Could you check a few things on this model? Use its own coordinates, in mm. A direction names the side the tool comes from. Round coordinates to 2 decimals unless told otherwise and drop trailing zeros. Write each loop counter-clockwise with the first axis right and the second up, starting at its lowest first coordinate (ties: lowest second). Pieces come first, ordered by that corner, then holes. Notation, with made-up numbers: (35, 40) - (71, 40) arc R12 cw to (71, 46) - close; hole circle Ø9 at (-12.5, -7). An arc over 180 degrees is marked (long way). Put each result on its own line as item: value.
from build123d import *

# Parameters (mm, degrees)
F0_R     = 3
F0_R_2   = 5.25
F1_DEPTH = 2


with BuildPart() as f1:
    # F0 (on Top) → F1 (new body)
    with BuildSketch(Plane.XY):
        with BuildLine():
            Line((-106.994636, 73.57139), (-148.369657, 73.57139))
            ThreePointArc((-148.369657, 73.57139), (-171.369657, 19.821374), (-148.369657, -33.928643))
            Line((-148.369657, -33.928643), (-106.994636, -33.928643))
            ThreePointArc((-106.994636, -33.928643), (-97.994636, -30.928643), (-88.994636, -33.928643))
            Line((-88.994636, -33.928643), (-47.619614, -33.928643))
            ThreePointArc((-47.619614, -33.928643), (-24.619614, 19.821374), (-47.619614, 73.57139))
            Line((-47.619614, 73.57139), (-88.994636, 73.57139))
            ThreePointArc((-88.994636, 73.57139), (-97.994636, 70.57139), (-106.994636, 73.57139))
        make_face()
        with Locations((-144.276634, -8.428643)):
            Circle(F0_R, mode=Mode.SUBTRACT)
        with Locations((-127.869657, 19.821374)):
            Circle(F0_R_2, mode=Mode.SUBTRACT)
        with Locations((-68.119614, 19.821374)):
            Circle(F0_R_2, mode=Mode.SUBTRACT)
        with BuildLine():
            Line((-123.994636, 30.821374), (-123.994636, 57.321374))
            Line((-123.994636, 57.321374), (-71.994636, 57.321374))
            Line((-71.994636, 57.321374), (-71.994636, 30.821374))
            Line((-71.994636, 30.821374), (-77.983549, 27.821374))
            ThreePointArc((-77.983549, 27.821374), (-77.149435, 23.859964), (-76.869614, 19.821374))
            ThreePointArc((-76.869614, 19.821374), (-77.149435, 15.782783), (-77.983549, 11.821374))
            Line((-77.983549, 11.821374), (-71.994636, 8.821374))
            Line((-71.994636, 8.821374), (-71.994636, -17.678626))
            Line((-71.994636, -17.678626), (-123.994636, -17.678626))
            Line((-123.994636, -17.678626), (-123.994636, 8.821374))
            Line((-123.994636, 8.821374), (-118.005723, 11.821374))
            ThreePointArc((-118.005723, 11.821374), (-118.839837, 15.782783), (-119.119657, 19.821374))
            ThreePointArc((-119.119657, 19.821374), (-118.839837, 23.859964), (-118.005723, 27.821374))
            Line((-118.005723, 27.821374), (-123.994636, 30.821374))
        make_face(mode=Mode.SUBTRACT)
        with Locations((-144.276634, 48.07139)):
            Circle(F0_R, mode=Mode.SUBTRACT)
    extrude(amount=F1_DEPTH)


solid = f1.part
(1) Imagine slicing it at C-C, the plane z = 0.5. List the corners of the cut face in (x, y) for me.
Values found:
outline: (-148.37, -33.93) - (-106.99, -33.93) arc R15 cw to (-88.99, -33.93) - (-47.62, -33.93) arc R74.31 ccw to (-47.62, 73.57) - (-88.99, 73.57) arc R15 cw to (-106.99, 73.57) - (-148.37, 73.57) arc R74.31 ccw to start; hole circle Ø6 at (-144.28, -8.43); hole circle Ø6 at (-144.28, 48.07); hole circle Ø10.5 at (-127.87, 19.82); hole (-123.99, -17.68) - (-71.99, -17.68) - (-71.99, 8.82) - (-77.98, 11.82) arc R29.28 ccw to (-76.87, 19.82) arc R29.28 ccw to (-77.98, 27.82) - (-71.99, 30.82) - (-71.99, 57.32) - (-123.99, 57.32) - (-123.99, 30.82) - (-118.01, 27.82) arc R29.28 ccw to (-119.12, 19.82) arc R29.28 ccw to (-118.01, 11.82) - (-123.99, 8.82) - close; hole circle Ø10.5 at (-68.12, 19.82)
(2) Please list where these lines run through material, in increasing order: probe 1 along Y at (x, z) = (-86.5, 1.3); probe 2 along X at (y, z) = (15, 1.2); probe 3 along X at (y, z) = (-8, 1.35). Write a range as from..to.
Values found:
probe 1: y = -33.93..-17.68, 57.32..73.57
probe 2: x = -171.21..-129.95, -125.79..-118.72, -77.27..-70.2, -66.04..-24.78
probe 3: x = -165.96..-147.25, -141.31..-123.99, -71.99..-30.02
(3) Imagine slicing it at A-A, the plane x = -80. List the corners of the cut face in (y, z) for me, then the cut area to 3 significant figures.
Values found:
outline: (-33.93, 0) - (-17.68, 0) - (-17.68, 2) - (-33.93, 2) - close; (57.32, 0) - (73.57, 0) - (73.57, 2) - (57.32, 2) - close
area: 65.0 mm^2
(4) For faces 1 (the face through (-66, 9, 0)), 2 (the face through (-120.96, 29.3, 0.99)), which set-ups out of +Z, -Z, +X, -X, +Y, -Y let a thin tool reach every point of the face, with its end or its side?
Values found:
face 1: -Z, +X, -X, +Y, -Y
face 2: +Z, -Z
(5) Imagine slicing it at D-D, the plane x = -157.5. List the corners of the cut face in (y, z) for me, then the cut area to 3 significant figures.
Values found:
outline: (-23.41, 0) - (63.05, 0) - (63.05, 2) - (-23.41, 2) - close
area: 173 mm^2
(6) If we mould it in two halves opening along X, with no side actions, what happens to faces 3 (the face through (-133.115, 20.052, 0.986)), 4 (the face through (-66, 9, 2)), 5 (the face through (-74.95, 29.34, 0.99)), 6 (the face through (-24.624, 18.98, 0.986))? For each: pulls with the +X half, pulls with the -X half, needs draft (parallel to the pull), parting line crosses it, or undercut.
Values found:
face 3: undercut
face 4: needs draft
face 5: undercut
face 6: pulls with the +X half
(7) Imagine slicing it at B-B, the plane y = 40. List the corners of the cut face in (x, z) for me.
Values found:
outline: (-168.58, 0) - (-123.99, 0) - (-123.99, 2) - (-168.58, 2) - close; (-71.99, 0) - (-27.41, 0) - (-27.41, 2) - (-71.99, 2) - close
(8) I'm going to push flat-ended pins straight in: pin 1 (12 mm diameter, centred on x = -127.87, y = 19.82, fed in from +Z); pin 2 (0.6 mm diameter, centred on y = -8, z = 1, fed in from +X); pin 3 (0.6 mm diameter, centred on x = -100, z = 1, fed in from +Y); pin 4 (1 mm diameter, centred on x = -42.5, z = 1.5, fed in from +Y). Where does each tip first touch, or does it pass through?
Values found:
pin 1: stops at z = 2
pin 2: stops at x = -29.9
pin 3: stops at y = 70.75
pin 4: stops at y = 68.75
